```python
from build123d import *

# Parameters (mm, degrees)
F0_R      = 10
F0_R_2    = 5
F1_DEPTH  = 30
F2_R      = 29
F2_R_2    = 10
F3_DEPTH  = 30
F5_DEPTH  = 30.001
F6_R      = 8
F7_R      = 1
F8_T      = -0.8
F9_DEPTH  = 25
F10_R     = 5.8
F10_R_2   = 5
F11_DEPTH = 30
F12_SIZE  = 1


with BuildPart() as f1:
    # F0 (on Front) → F1 (new body)
    with BuildSketch(Plane.XZ):
        Circle(F0_R)
        Circle(F0_R_2, mode=Mode.SUBTRACT)
    extrude(amount=F1_DEPTH)

    # F2 (on face) → F3 (join, through all)
    with BuildSketch(Plane.XZ.offset(30)):
        Circle(F2_R)
        Circle(F2_R_2, mode=Mode.SUBTRACT)
    extrude(amount=-F3_DEPTH)

    # F4 (on face) → F5 (cut, through all)
    with BuildSketch(Plane.XZ.offset(30)):
        with BuildLine():
            ThreePointArc((-9.5393920142, -3), (-10, 0), (-9.5393920142, 3))
            Line((-9.5393920142, 3), (-32.1717076004, 3))
            Line((-32.1717076004, 3), (-32.1717076004, -3))
            Line((-32.1717076004, -3), (-9.5393920142, -3))
        make_face()
        with BuildLine():
            Line((-3, -33.598061651), (3, -33.598061651))
            Line((3, -33.598061651), (3, -9.5393920142))
            ThreePointArc((3, -9.5393920142), (0, -10), (-3, -9.5393920142))
            Line((-3, -9.5393920142), (-3, -33.598061651))
        make_face()
        with BuildLine():
            Line((3, 9.5393920142), (3, 33.598061651))
            Line((3, 33.598061651), (-3, 33.598061651))
            Line((-3, 33.598061651), (-3, 9.5393920142))
            ThreePointArc((-3, 9.5393920142), (0, 10), (3, 9.5393920142))
        make_face()
        with BuildLine():
            Line((9.5393920142, -3), (32.1717076004, -3))
            Line((32.1717076004, -3), (32.1717076004, 3))
            Line((32.1717076004, 3), (9.5393920142, 3))
            ThreePointArc((9.5393920142, 3), (10, 0), (9.5393920142, -3))
        make_face()
    extrude(amount=-F5_DEPTH, mode=Mode.SUBTRACT)

    # F6
    f6_edges = [f1.edges().sort_by_distance(p)[0] for p in [
        (-3, -15, 28.84441),
        (-28.84441, -15, 3),
        (-28.84441, -15, -3),
        (3, -15, 28.84441),
        (-3, -15, -28.84441),
        (3, -15, -28.84441),
        (28.84441, -15, -3),
        (28.84441, -15, 3),
    ]]
    fillet(f6_edges, radius=F6_R)

    # F7
    f7_edges = [f1.edges().sort_by_distance(p)[0] for p in [
        (-9.539392, -15, 3),
        (-9.539392, -15, -3),
        (-3, -15, -9.539392),
        (3, -15, -9.539392),
        (9.539392, -15, 3),
        (9.539392, -15, -3),
        (-3, -15, 9.539392),
        (3, -15, 9.539392),
    ]]
    fillet(f7_edges, radius=F7_R)

    # F8
    f8_openings = [f1.faces().sort_by_distance(p)[0] for p in [
        (14.352599, -30, 3.732239),
    ]]
    offset(amount=F8_T, openings=f8_openings)

    # F9 (cut): faces of the model
    f9_faces = [f1.faces().sort_by_distance(p)[0] for p in [
        (14.3525988232, -0.8, 4.5096111786),
        (14.3525988232, -0.8, 4.5096111786),
        (14.3525988232, -0.8, 4.5096111786),
        (14.3525988232, -0.8, 4.5096111786),
    ]]
    extrude(f9_faces, amount=-F9_DEPTH, mode=Mode.SUBTRACT)

    # F10 (on face) → F11 (join, through all)
    with BuildSketch(Plane.XZ.offset(30)):
        with BuildLine():
            ThreePointArc((9.0466559275, 1.6727272727), (9.083408006, 2.4856530923), (9.4744050932, 3.1993199482))
            ThreePointArc((9.4744050932, 3.1993199482), (7.0710678119, 7.0710678119), (3.1993199482, 9.4744050932))
            ThreePointArc((3.1993199482, 9.4744050932), (2.4856530923, 9.083408006), (1.6727272727, 9.0466559275))
            ThreePointArc((1.6727272727, 9.0466559275), (0, 9.2), (-1.6727272727, 9.0466559275))
            ThreePointArc((-1.6727272727, 9.0466559275), (-2.4856530923, 9.083408006), (-3.1993199482, 9.4744050932))
            ThreePointArc((-3.1993199482, 9.4744050932), (-7.0710678119, 7.0710678119), (-9.4744050932, 3.1993199482))
            ThreePointArc((-9.4744050932, 3.1993199482), (-9.083408006, 2.4856530923), (-9.0466559275, 1.6727272727))
            ThreePointArc((-9.0466559275, 1.6727272727), (-9.2, 0), (-9.0466559275, -1.6727272727))
            ThreePointArc((-9.0466559275, -1.6727272727), (-9.083408006, -2.4856530923), (-9.4744050932, -3.1993199482))
            ThreePointArc((-9.4744050932, -3.1993199482), (-7.0710678119, -7.0710678119), (-3.1993199482, -9.4744050932))
            ThreePointArc((-3.1993199482, -9.4744050932), (-2.4856530923, -9.083408006), (-1.6727272727, -9.0466559275))
            ThreePointArc((-1.6727272727, -9.0466559275), (0, -9.2), (1.6727272727, -9.0466559275))
            ThreePointArc((1.6727272727, -9.0466559275), (2.4856530923, -9.083408006), (3.1993199482, -9.4744050932))
            ThreePointArc((3.1993199482, -9.4744050932), (7.0710678119, -7.0710678119), (9.4744050932, -3.1993199482))
            ThreePointArc((9.4744050932, -3.1993199482), (9.083408006, -2.4856530923), (9.0466559275, -1.6727272727))
            ThreePointArc((9.0466559275, -1.6727272727), (9.2, 0), (9.0466559275, 1.6727272727))
        make_face()
        Circle(F10_R, mode=Mode.SUBTRACT)
        Circle(F10_R)
        Circle(F10_R_2, mode=Mode.SUBTRACT)
    extrude(amount=-F11_DEPTH)

    # F12
    f12_edges = [f1.edges().sort_by_distance(p)[0] for p in [
        (5, -15, 0),
        (-5, 0, 0),
        (-5, -30, 0),
    ]]
    chamfer(f12_edges, length=F12_SIZE)


solid = f1.part
```
The listing builds one solid part. Answer for the finished solid, in the listing's coordinates (mm). A direction names the side the tool comes from. Coordinates: 2 decimals unless noted, no trailing zeros. Loops run counter-clockwise (first coordinate to the right, second up) from the corner with the lowest first, then second, coordinate; pieces in that order, holes last. Notation, with made-up numbers: (65, -33.5) - (101, -33.5) arc R17 cw to (101, -27.5) - close; hole circle Ø7 at (-16.5, 50.25). An arc over 180 degrees is marked (long way). Use a Markdown table: item, result. Add a question column.
1) The part is cut by section C-C, the plane x = 11.5. Give the vertices of the cut face in (y, z).
2) The part is cut by section A-A, the plane x = 0. Give the vertices of the cut face in (y, z).
3) The part is cut by section D-D, the plane z = 16.5. Give the vertices of the cut face in (x, y), and give its area (3 significant figures).
4) Given pin 1 (9 mm diameter, centred on x = 0, z = 0, fed in from -Y); pin 2 (5.5 mm diameter, centred on y = -8, z = 15.5, fed in from +X); pin 3 (3 mm diameter, centred on y = -14.5, z = 14, fed in from -X); pin 4 (2 mm diameter, centred on x = 15, y = -10, fed in from -Z), each flat-ended and moving along its own axis, determine where each tip first touches the part or whether it passes through.
5) Find the intervals of material crossed by line 1 (X direction, y = -17.75, z = -11); line 2 (Z direction, x = 0, y = -13), in increasing order.
6) For faces 1 (the flat face through (3.8, -15, 14)), 2 (the flat face through (-3, -15, -14)), 3 (the cylindrical face through (20, -15, -21)), 4 (the flat face through (-14, -15, 3)), determine the directions among +Z, -Z, +X, -X, +Y, -Y from which every point of the face is accessible in a straight line to the end or side of a thin tool.
7) The mould has two halves that part along Z. Classify faces 5 (the flat face through (-6, -30, -2)), 6 (the cylindrical face through (-20, -15, 21)), 7 (the cylindrical face through (19.87, -15.21, -20.01)), 8 (the cylindrical face through (-6.99, -15.21, -24.81)): released by +Z, released by -Z, zero draft, split by the parting line, or undercut.
8) The part is cut by section B-B, the plane z = 0. Give the vertices of the cut face in (x, y).
Here are the results:
| question | item | result |
|---|---|---|
| 1 | outline | (-30, -25.87) - (0, -25.87) - (0, -25.07) - (-30, -25.07) - close; (-30, -3.8) - (0, -3.8) - (0, -3) - (-30, -3) - close; (-30, 3) - (0, 3) - (0, 3.8) - (-30, 3.8) - close; (-30, 25.07) - (0, 25.07) - (0, 25.87) - (-30, 25.87) - close |
| 2 | outline | (-30, -10) - (0, -10) - (0, -6) - (-1, -5) - (-29, -5) - (-30, -6) - close; (-30, 6) - (-29, 5) - (-1, 5) - (0, 6) - (0, 10) - (-30, 10) - close |
| 3 | outline | (-23.85, -30) - (-22.87, -30) - (-22.87, 0) - (-23.85, 0) - close; (-3.8, -30) - (-3, -30) - (-3, 0) - (-3.8, 0) - close; (3, -30) - (3.8, -30) - (3.8, 0) - (3, 0) - close; (22.87, -30) - (23.85, -30) - (23.85, 0) - (22.87, 0) - close |
| 3 | area | 107 mm^2 |
| 4 | pin 1 | passes through |
| 4 | pin 2 | stops at x = 25.69 |
| 4 | pin 3 | stops at x = -25.75 |
| 4 | pin 4 | stops at z = -25.3 |
| 5 | line 1 | x = -25.89 to -25.09, -3.8 to -3, 3 to 3.8, 25.09 to 25.89 |
| 5 | line 2 | z = -10 to -5, 5 to 10 |
| 6 | face 1 | +Y, -Y |
| 6 | face 2 | -Z, +Y, -Y |
| 6 | face 3 | -Z, +X, +Y, -Y |
| 6 | face 4 | -X, +Y, -Y |
| 7 | face 5 | zero draft |
| 7 | face 6 | released by +Z |
| 7 | face 7 | undercut |
| 7 | face 8 | released by -Z |
| 8 | outline | (-10, -30) - (-6, -30) - (-5, -29) - (-5, -1) - (-6, 0) - (-10, 0) - close; (5, -29) - (6, -30) - (10, -30) - (10, 0) - (6, 0) - (5, -1) - close |
